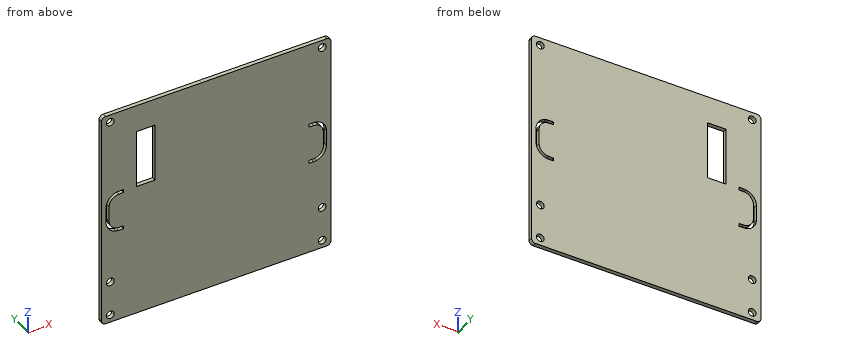
from build123d import *

# Parameters (mm, degrees)
SKETCH1_R           = 3
SKETCH1_W           = 14.2494
SKETCH1_H           = 44.671382498
BOSS_EXTRUDE1_DEPTH = 3.175
FILLET1_R           = 3.175


with BuildPart() as part:
    # Sketch1 → Boss-Extrude1 (new body)
    with BuildSketch(Plane(origin=(0, 0, 0), x_dir=(1, 0, 0), z_dir=(0, 1, 0))):
        Polygon((16.960672162, 168.629876359), (160.039327838, 168.629876359), (177, 168.629876359), (177, 0), (160.039327838, 0), (16.960672162, 0), (0, 0), (0, 168.629876359), align=None)
        with Locations((6.800672162, 162.669204197)):
            Circle(SKETCH1_R, mode=Mode.SUBTRACT)
        with Locations((6.800672162, 135.969204197)):
            Circle(SKETCH1_R, mode=Mode.SUBTRACT)
        with Locations((170.199327838, 162.669204197)):
            Circle(SKETCH1_R, mode=Mode.SUBTRACT)
        with Locations((170.199327838, 135.969204197)):
            Circle(SKETCH1_R, mode=Mode.SUBTRACT)
        with Locations((6.800672162, 5.96493818)):
            Circle(SKETCH1_R, mode=Mode.SUBTRACT)
        with Locations((170.199327838, 5.96493818)):
            Circle(SKETCH1_R, mode=Mode.SUBTRACT)
        with Locations((34, 43.470295491)):
            Rectangle(SKETCH1_W, SKETCH1_H, mode=Mode.SUBTRACT)
        with BuildLine():
            Line((16.951048024, 64.540050733), (16.991793389, 66.874351095))
            Line((16.991793389, 66.874351095), (13.367278288, 66.937617241))
            ThreePointArc((13.367278288, 66.937617241), (8.075887225, 69.210978252), (5.895219965, 74.541239031))
            Line((5.895219965, 74.541239031), (5.895219965, 86.398551951))
            ThreePointArc((5.895219965, 86.398551951), (8.075887225, 91.72881273), (13.367278288, 94.00217374))
            Line((13.367278288, 94.00217374), (16.987373531, 94.065362738))
            Line((16.987373531, 94.065362738), (16.946445409, 96.410133308))
            Line((16.946445409, 96.410133308), (13.326350165, 96.34694431))
            ThreePointArc((13.326350165, 96.34694431), (12.377781101, 96.284971401), (11.439455037, 96.132760663))
            Line((11.439455037, 96.132760663), (11.375913148, 96.152499099))
            ThreePointArc((11.375913148, 96.152499099), (5.72648647, 92.661436057), (3.517453736, 86.398551951))
            Line((3.517453736, 86.398551951), (3.517453736, 74.541239031))
            ThreePointArc((3.517453736, 74.541239031), (5.726486031, 68.278355625), (11.375911736, 64.787292544))
            Line((11.375911736, 64.787292544), (11.459759836, 64.8134536))
            ThreePointArc((11.459759836, 64.8134536), (12.38817048, 64.664183621), (13.326532399, 64.603316889))
            Line((13.326532399, 64.603316889), (16.951048024, 64.540050733))
        make_face(mode=Mode.SUBTRACT)
        with BuildLine():
            Line((160.012549311, 66.878848625), (160.053371832, 64.540127941))
            Line((160.053371832, 64.540127941), (163.673466588, 64.60331693))
            ThreePointArc((163.673466588, 64.60331693), (164.611836733, 64.664184588), (165.540255354, 64.81345704))
            Line((165.540255354, 64.81345704), (165.624086371, 64.787291495))
            ThreePointArc((165.624086371, 64.787291495), (171.273513049, 68.278354537), (173.482545784, 74.541238643))
            Line((173.482545784, 74.541238643), (173.482545784, 86.398551563))
            ThreePointArc((173.482545784, 86.398551563), (171.273513446, 92.661435036), (165.624087648, 96.152498114))
            Line((165.624087648, 96.152498114), (165.560531376, 96.132763539))
            ThreePointArc((165.560531376, 96.132763539), (164.622211999, 96.284972184), (163.673649835, 96.34694431))
            Line((163.673649835, 96.34694431), (160.04913421, 96.410210466))
            Line((160.04913421, 96.410210466), (160.008128929, 94.061019514))
            Line((160.008128929, 94.061019514), (163.632644554, 93.997753359))
            ThreePointArc((163.632644554, 93.997753359), (168.920959456, 91.725713971), (171.10035898, 86.398551951))
            Line((171.10035898, 86.398551951), (171.10035898, 74.541239031))
            ThreePointArc((171.10035898, 74.541239031), (168.920959456, 69.21407701), (163.632644554, 66.942037623))
            Line((163.632644554, 66.942037623), (160.012549311, 66.878848625))
        make_face(mode=Mode.SUBTRACT)
    extrude(amount=BOSS_EXTRUDE1_DEPTH)

    # Fillet1
    fillet1_edges = [part.edges().sort_by_distance(p)[0] for p in [
        (0, 1.5875, 0),
        (0, 1.5875, -168.629876359),
        (177, 1.5875, -168.629876359),
        (177, 1.5875, 0),
    ]]
    fillet(fillet1_edges, radius=FILLET1_R)


solid = part.part
Can you work these out from the model? Positions are in its coordinate system, mm. Coordinates: 2 decimals unless noted, no trailing zeros. Write each loop counter-clockwise with the first axis right and the second up, starting at its lowest first coordinate (ties: lowest second). Pieces come first, ordered by that corner, then holes. Notation, with made-up numbers: (81.25, 39) -> (131.25, 39) arc R23 cw to (131.25, 52) -> close; hole circle Ø11 at (5.5, -36.75). An arc over 180 degrees is marked (long way). Answer as CSV lines item,"result".
1) If we section it at A-A on z = -46: Please give me the cut outline in (x, y) (3 decimals), then the cut area to 3 significant figures.
Check result:
outline,"(0, 0) -> (26.875, 0) -> (26.875, 3.175) -> (0, 3.175) -> close; (41.125, 0) -> (177, 0) -> (177, 3.175) -> (41.125, 3.175) -> close"
area,"517 mm²"
2) If we section it at B-B on z = -92: Please give me the cut outline in (x, y) (3 decimals), then the cut area to 3 significant figures.
Check result:
outline,"(0, 0) -> (5.237, 0) -> (5.237, 3.175) -> (0, 3.175) -> close; (8.356, 0) -> (168.637, 0) -> (168.637, 3.175) -> (8.356, 3.175) -> close; (171.763, 0) -> (177, 0) -> (177, 3.175) -> (171.763, 3.175) -> close"
area,"542 mm²"
3) If I drill on line 1 (X direction, y = 2.4, z = -24.5); line 2 (X direction, y = 1.15, z = -7); line 3 (Z direction, x = 36.5, y = 0.95), over which ranges is the centre line in solid material (lowest first)? Write a range as from..to.
Check result:
line 1,"0..26.88, 41.12..177"
line 2,"0..3.98, 9.62..167.38, 173.02..177"
line 3,"-168.63..-65.81, -21.13..0"
4) If we section it at C-C on y = 0.5: Count the separate pieces of the cut face and the enclosed holes in it, then the cut area to 3 significant figures.
Check result:
separate pieces,"1"
enclosed holes,"9"
area,"28,800 mm²"
